Geometry check sheet. Reference: the model listing, model coordinates, mm. A direction names the side the tool comes from. Round coordinates to 2 decimals unless told otherwise and drop trailing zeros. Order: outer loops, then holes, each group sorted by start corner. A loop starts at its lowest first (then second) coordinate and runs counter-clockwise, first axis right, second up. Notation, with made-up numbers: (19.5, 70.25) - (57.5, 70.25) arc R28 ccw to (57.5, 106.25) - close; hole circle Ø10 at (47, 34.5). An arc over 180 degrees is marked (long way). Use a Markdown table: item, result. Add a question column.
(1) Mould release check, pull along Y, two halves, no side actions. Record for faces 4 (the face through (3.22, 3.29, 1.97)), 5 (the face through (6, 5, 4)): released by +Y, released by -Y, zero draft, split by the parting line, or undercut.
(2) Section check D-D on z = 3. Record the boundary of the cut face in (x, y), then the cut area to 3 significant figures.
(3) Gauge pin test, flat ends, axial feed: P1, Ø4, axis at y = 10, z = 1, coming from the -X side; P2, Ø1, axis at x = 9.5, z = -1.5, coming from the +Y side; P3, Ø4, axis at y = 1, z = -1.5, coming from the -X side. Record the tip position at first contact, or that the pin passes through.
(4) Section check C-C on x = 13.35. Record the boundary of the cut face in (y, z), then the cut area to 3 significant figures.
(5) Thickness scan on line 1 along X through (y, z) = (4, 2.75); line 2 along X through (y, z) = (7, -2.1); line 3 along X through (y, z) = (10.5, 3). Record the ranges inside material, lowest first. Write a range as [from, to].
(6) Access from +Z, -Z, +X, -X, +Y, -Y to the whole of each face (thin tool, end or side, straight path). Record for faces 1 (the face through (7, 8, 1.6)), 2 (the face through (14.08, 11.78, -1.48)), 3 (the face through (8, 0, -3)).
(7) Section check A-A on z = 1.25. Record the boundary of the cut face in (x, y).
(8) Section check B-B on x = 8.1. Record the boundary of the cut face in (y, z), then the cut area to 3 significant figures.
```python
from build123d import *
from build123d.topology import SkipClean

# Parameters (mm, degrees)
SKETCH1_R           = 0.8
BOSS_EXTRUDE1_DEPTH = 4
CUT_EXTRUDE1_DEPTH  = 2.4
SKETCH3_R           = 1.3
CUT_EXTRUDE2_DEPTH  = 4
BOSS_EXTRUDE2_DEPTH = 3


with BuildPart() as part:
    # Sketch1 → Boss-Extrude1 (new body)
    with BuildSketch(Plane.XY):
        with BuildLine():
            Line((0, 12.5), (16.2, 12.5))
            ThreePointArc((16.2, 12.5), (8.1, -2.790812019), (0, 12.5))
        make_face()
        with Locations((2.85, 10)):
            Circle(SKETCH1_R, mode=Mode.SUBTRACT)
        with Locations(Location((13.35, 10, 0), (0, 0, 180))):
            Circle(SKETCH1_R, mode=Mode.SUBTRACT)
        with Locations(Location((13.35, 4, 0), (0, 0, 180))):
            Circle(SKETCH1_R, mode=Mode.SUBTRACT)
        with Locations((2.85, 4)):
            Circle(SKETCH1_R, mode=Mode.SUBTRACT)
    extrude(amount=BOSS_EXTRUDE1_DEPTH)

    # Sketch2 → Cut-Extrude1 (cut)
    with BuildSketch(Plane.XY.offset(4)):
        Polygon((10.813546265, 7), (9.456773133, 9.35), (6.743226867, 9.35), (5.386453735, 7), (6.743226867, 4.65), (9.456773133, 4.65), align=None)
    extrude(amount=-CUT_EXTRUDE1_DEPTH, mode=Mode.SUBTRACT)

    # Sketch3 → Cut-Extrude2 (cut)
    with BuildSketch(Plane.XY.offset(4)):
        with Locations((8.1, 7)):
            Circle(SKETCH3_R)
    extrude(amount=-CUT_EXTRUDE2_DEPTH, mode=Mode.SUBTRACT)

    # Sketch4 → Boss-Extrude2 (add)
    with SkipClean():  # the faces are left unmerged after this step: merging them gives an invalid solid
        with BuildSketch(Plane.XY):
            with BuildLine():
                Line((16.2, 12.5), (15.362063339, 12.5))
                ThreePointArc((15.362063339, 12.5), (14.070641831, 11.763040292), (14.048187812, 10.276307316))
                ThreePointArc((14.048187812, 10.276307316), (8.1, 0.209187981), (2.151812188, 10.276307316))
                ThreePointArc((2.151812188, 10.276307316), (2.129358169, 11.763040292), (0.837936661, 12.5))
                Line((0.837936661, 12.5), (0, 12.5))
                ThreePointArc((0, 12.5), (8.1, -2.790812019), (16.2, 12.5))
            make_face()
        extrude(amount=-BOSS_EXTRUDE2_DEPTH)


solid = part.part
```
Check sheet entries:
| question | item | result |
|---|---|---|
| 1 | face 4 | undercut |
| 1 | face 5 | zero draft |
| 2 | outline | (0, 12.5) arc R9.79 ccw (long way) to (16.2, 12.5) - close; hole circle Ø1.6 at (2.85, 4); hole circle Ø1.6 at (2.85, 10); hole (5.39, 7) - (6.74, 4.65) - (9.46, 4.65) - (10.81, 7) - (9.46, 9.35) - (6.74, 9.35) - close; hole circle Ø1.6 at (13.35, 4); hole circle Ø1.6 at (13.35, 10) |
| 2 | area | 225 mm2 |
| 3 | P1 | stops at x = -1.64 |
| 3 | P2 | stops at y = 0.48 |
| 3 | P3 | stops at x = -0.84 |
| 4 | outline | (-1.26, -3) - (2.69, -3) - (2.69, 0) - (3.2, 0) - (3.2, 4) - (-1.26, 4) - close; (4.8, 0) - (9.2, 0) - (9.2, 4) - (4.8, 4) - close; (10.8, 0) - (12.5, 0) - (12.5, 4) - (10.8, 4) - close |
| 4 | area | 54.1 mm2 |
| 5 | line 1 | x = [-1.22, 2.05], [3.65, 12.55], [14.15, 17.42] |
| 5 | line 2 | x = [-1.69, 1.31], [14.89, 17.89] |
| 5 | line 3 | x = [-1.04, 2.23], [3.47, 12.73], [13.97, 17.24] |
| 6 | face 1 | +Z |
| 6 | face 2 | -Z |
| 6 | face 3 | -Z, +X, -X, +Y, -Y |
| 7 | outline | (0, 12.5) arc R9.79 ccw (long way) to (16.2, 12.5) - close; hole circle Ø1.6 at (2.85, 4); hole circle Ø1.6 at (2.85, 10); hole circle Ø2.6 at (8.1, 7); hole circle Ø1.6 at (13.35, 4); hole circle Ø1.6 at (13.35, 10) |
| 8 | outline | (-2.79, -3) - (0.21, -3) - (0.21, 0) - (5.7, 0) - (5.7, 1.6) - (4.65, 1.6) - (4.65, 4) - (-2.79, 4) - close; (8.3, 0) - (12.5, 0) - (12.5, 4) - (9.35, 4) - (9.35, 1.6) - (8.3, 1.6) - close |
| 8 | area | 54.7 mm2 |
